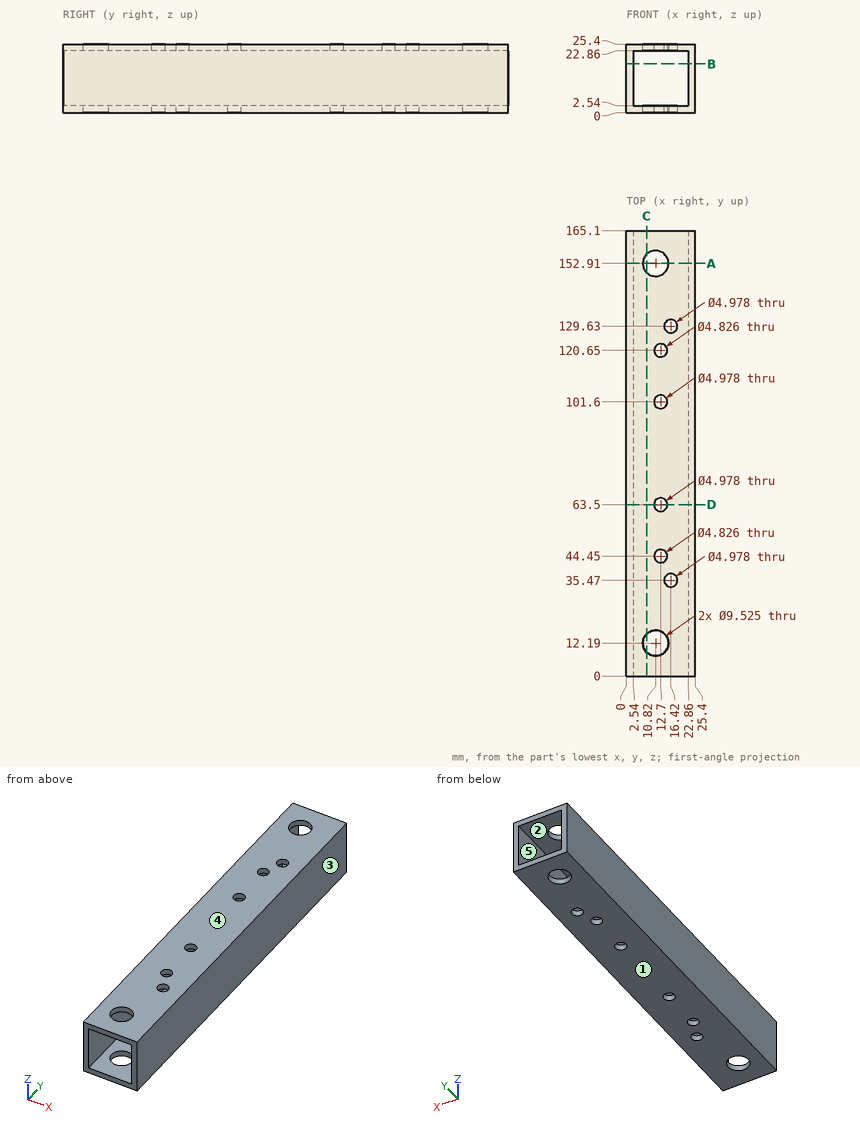
Study the drawing (mm; zero at the part's minimum x, y, z) and answer. A direction names the side the tool comes from. Coordinates: 2 decimals unless noted, no trailing zeros. Write each loop counter-clockwise with the first axis right and the second up, starting at its lowest first coordinate (ties: lowest second). Pieces come first, ordered by that corner, then holes. Notation, with made-up numbers: M 63.25,86.5 L 98.25,86.5 A31 cw 98.25,117.5 Z; hole C -26.75,6.25 d7. An arc over 180 degrees is marked long. Write each question's results on one line, items separated by ' | '.
Item 1: For a pull along X with two mould halves and no side action, classify the marked faces 3, 4 and 5 as released by +X, released by -X, zero draft, split by the parting line, or undercut.
Answer below:
face 3: released by +X | face 4: zero draft | face 5: undercut
Item 2: The part is cut by section A-A on y = 152.91. Determine the outline of the cut face in (x, z), and give its area (3 significant figures).
Answer below:
outline: M 0,0 L 6.06,0 L 6.06,2.54 L 2.54,2.54 L 2.54,22.86 L 6.06,22.86 L 6.06,25.4 L 0,25.4 Z; M 15.58,0 L 25.4,0 L 25.4,25.4 L 15.58,25.4 L 15.58,22.86 L 22.86,22.86 L 22.86,2.54 L 15.58,2.54 Z | area: 184 mm2
Item 3: Which of the six approach directions +Z, -Z, +X, -X, +Y, -Y give full straight-line access (tool end or side, diameter ignored) to the marked faces 1 and 2?
Answer below:
face 1: -Z, +X, -X, +Y, -Y | face 2: +Y, -Y
Item 4: The part is cut by section C-C on x = 7.5. Determine the outline of the cut face in (y, z).
Answer below:
outline: M 0,0 L 8.78,0 L 8.78,2.54 L 0,2.54 Z; M 0,22.86 L 8.78,22.86 L 8.78,25.4 L 0,25.4 Z; M 15.6,0 L 149.5,0 L 149.5,2.54 L 15.6,2.54 Z; M 15.6,22.86 L 149.5,22.86 L 149.5,25.4 L 15.6,25.4 Z; M 156.32,0 L 165.1,0 L 165.1,2.54 L 156.32,2.54 Z; M 156.32,22.86 L 165.1,22.86 L 165.1,25.4 L 156.32,25.4 Z
Item 5: Consider probe 1 along X at (y, z) = (12.19, 1); probe 2 along X at (y, z) = (26, 21.75). Determine where each line is inside the solid, lowest interval first. Write a range as [from, to].
Answer below:
probe 1: [0, 6.06], [15.58, 25.4] | probe 2: [0, 2.54], [22.86, 25.4]
Item 6: The part is cut by section B-B on z = 18. Determine the outline of the cut face in (x, y).
Answer below:
outline: M 0,0 L 2.54,0 L 2.54,165.1 L 0,165.1 Z; M 22.86,0 L 25.4,0 L 25.4,165.1 L 22.86,165.1 Z
Item 7: The part is cut by section D-D on y = 63.5. Determine the outline of the cut face in (x, z).
Answer below:
outline: M 0,0 L 10.21,0 L 10.21,2.54 L 2.54,2.54 L 2.54,22.86 L 10.21,22.86 L 10.21,25.4 L 0,25.4 Z; M 15.19,0 L 25.4,0 L 25.4,25.4 L 15.19,25.4 L 15.19,22.86 L 22.86,22.86 L 22.86,2.54 L 15.19,2.54 Z
